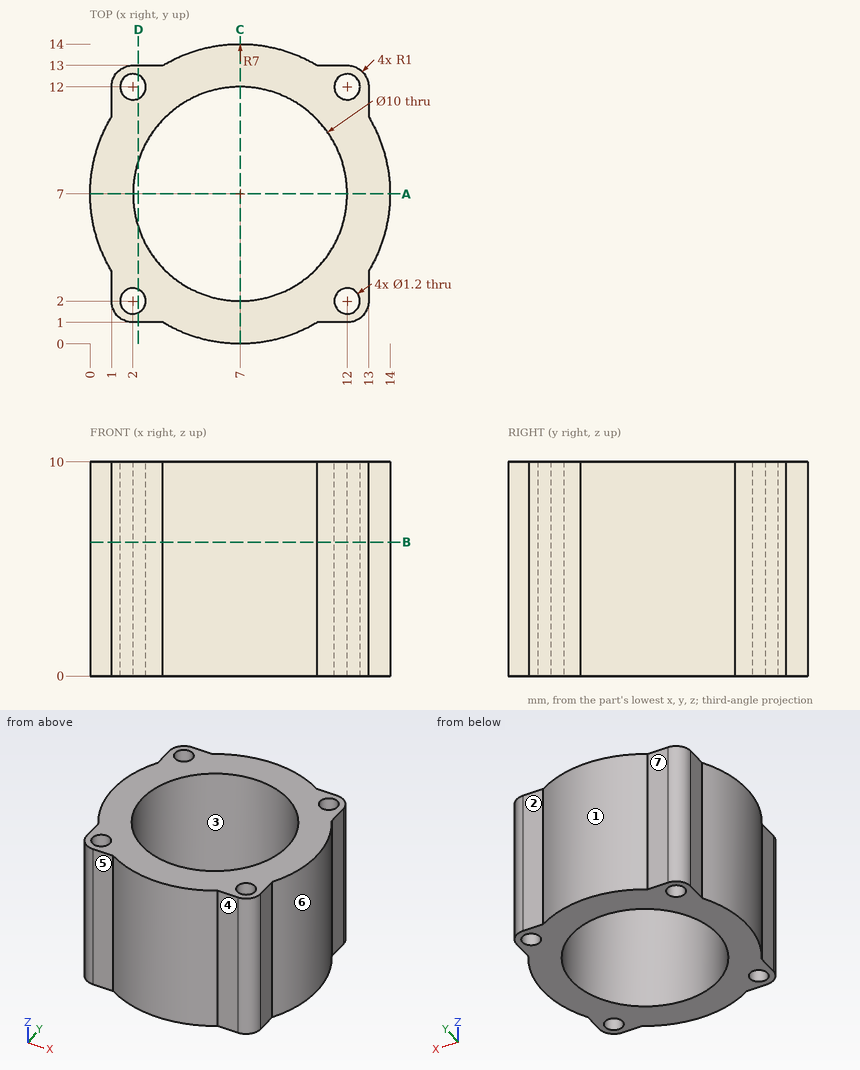
The drawing under review shows one solid part. Ordinate dimensions are in mm from its lowest x, y, z. A direction names the side the tool comes from. Round coordinates to 2 decimals unless told otherwise and drop trailing zeros. Write each loop counter-clockwise with the first axis right and the second up, starting at its lowest first coordinate (ties: lowest second). Pieces come first, ordered by that corner, then holes. Notation, with made-up numbers: (45.25, 83.25) -> (64.25, 83.25) arc R26 ccw to (64.25, 117.25) -> close; hole circle Ø5 at (63, 24). An arc over 180 degrees is marked (long way). Put each result on its own line as item: value.
Q1. Clearance check with flat-ended pins moving along their axes: pin 1 Ø1.1 at (x, z) = (11.5, 3) entering from +Y; pin 2 Ø0.7 at (x, y) = (2, 12) entering from +Z; pin 3 Ø4 at (x, z) = (4.5, 3) entering from -Y; pin 4 Ø1.5 at (x, z) = (3, 4.5) entering from -Y. State where each tip first meets the part, or that it passes through.
Determined:
pin 1: stops at y = 13
pin 2: passes through
pin 3: stops at y = 0.02
pin 4: stops at y = 0.8
Q2. To check wall thickness, follow L1, parallel to Y at x = 7, z = 2; L2, parallel to Y at x = 4.75, z = 3.75; L3, parallel to X at y = 2.5, z = 7.5. State the ranges of each line that lie inside material, in increasing order. Write a range as [from, to].
Determined:
L1: y = [0, 2], [12, 14]
L2: y = [0.37, 2.53], [11.47, 13.63]
L3: x = [1, 1.67], [2.33, 4.82], [9.18, 11.67], [12.33, 13]
Q3. The part is to be moulded in two halves that separate along X. For the marked faces 1, 2 and 3, say which applies: released by +X, released by -X, zero draft, split by the parting line, or undercut.
Determined:
face 1: split by the parting line
face 2: zero draft
face 3: undercut
Q4. Consider section D-D on x = 2.25. State the section outline as (y, z) points.
Determined:
outline: (1, 0) -> (1.45, 0) -> (1.45, 10) -> (1, 10) -> close; (2.55, 0) -> (5.44, 0) -> (5.44, 10) -> (2.55, 10) -> close; (8.56, 0) -> (11.45, 0) -> (11.45, 10) -> (8.56, 10) -> close; (12.55, 0) -> (13, 0) -> (13, 10) -> (12.55, 10) -> close
Q5. Consider section B-B on z = 6.25. State the section outline as (x, y) points.
Determined:
outline: (1, 2) arc R1 ccw to (2, 1) -> (3.39, 1) arc R7 ccw to (10.61, 1) -> (12, 1) arc R1 ccw to (13, 2) -> (13, 3.39) arc R7 ccw to (13, 10.61) -> (13, 12) arc R1 ccw to (12, 13) -> (10.61, 13) arc R7 ccw to (3.39, 13) -> (2, 13) arc R1 ccw to (1, 12) -> (1, 10.61) arc R7 ccw to (1, 3.39) -> close; hole circle Ø1.2 at (2, 2); hole circle Ø1.2 at (2, 12); hole circle Ø10 at (7, 7); hole circle Ø1.2 at (12, 2); hole circle Ø1.2 at (12, 12)
Q6. Consider section A-A on y = 7. State the section outline as (x, z) points.
Determined:
outline: (0, 0) -> (2, 0) -> (2, 10) -> (0, 10) -> close; (12, 0) -> (14, 0) -> (14, 10) -> (12, 10) -> close
Q7. Machinability: for the marked faces 4, 5, 6 and 7, which of the approach directions +Z, -Z, +X, -X, +Y, -Y give a long, thin tool a straight path to every point of the face, cutting with its end or side? Answer none if there is none.
Determined:
face 4: +Z, -Z, +X, -Y
face 5: +Z, -Z, -X, -Y
face 6: +Z, -Z, +X
face 7: +Z, -Z, -X, +Y
